```python
from build123d import *

# Parameters (mm, degrees)
F0_R     = 3.175
F1_DEPTH = 25.4
F2_R     = 2.38125
F3_DEPTH = 12.701
F4_SIZE2 = 0.79375
F4_SIZE  = 3.175


with BuildPart() as f1:
    # F0 (on Front) → F1 (new body)
    with BuildSketch(Plane.XZ):
        with BuildLine():
            ThreePointArc((6.35, 3.175), (3.175, -8.674261314), (11.849261314, 0))
            Line((11.849261314, 0), (228.6, 0))
            Line((228.6, 0), (228.6, 3.175))
            Line((228.6, 3.175), (6.35, 3.175))
        make_face()
        with Locations((6.35, -3.175)):
            Circle(F0_R, mode=Mode.SUBTRACT)
    extrude(amount=F1_DEPTH)

    # F2 (on face) → F3 (cut, through all)
    with BuildSketch(Plane.XY.offset(3.175)):
        with Locations((203.2, -12.7)):
            Circle(F2_R)
        with Locations((114.3, -12.7)):
            Circle(F2_R)
        with Locations((25.4, -12.7)):
            Circle(F2_R)
        Polygon((12.7, -8.382), (12.7, 5.4248190135), (-5.8604556464, 5.4248190135), (-5.8604556464, -32.8125189408), (12.7, -32.8125189408), (12.7, -16.764), (0, -16.764), (0, -8.382), align=None)
    extrude(amount=-F3_DEPTH, mode=Mode.SUBTRACT)

    # F4
    f4_edges = [f1.edges().sort_by_distance(p)[0] for p in [
        (120.65, -25.4, 0),
        (120.65, 0, 0),
        (228.6, -12.7, 0),
    ]]
    f4_side = f1.faces().sort_by_distance((120.570284, -12.699833, 0))[0]
    chamfer(f4_edges, length=F4_SIZE, length2=F4_SIZE2, reference=f4_side)


solid = f1.part
```
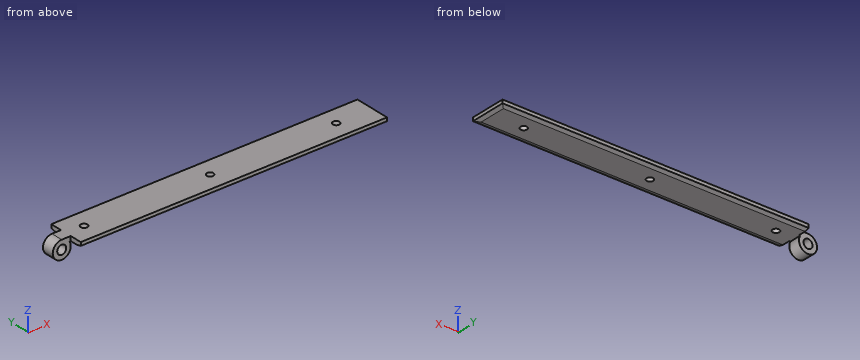
Geometry: final body of the model. Coordinates: model frame, mm. Coordinates: 2 decimals unless noted, no trailing zeros. Write each loop counter-clockwise with the first axis right and the second up, starting at its lowest first coordinate (ties: lowest second). Pieces come first, ordered by that corner, then holes. Notation, with made-up numbers: M 5.25,-23 L 48.25,-23 A16 ccw 48.25,4 Z; hole C 11,85.5 d3. An arc over 180 degrees is marked long. Answer as CSV lines item,"result". Start each with the question number.
Q1. Pin query (flat end, axial travel): P1, Ø7.5, axis at x = 6.35, z = -3.175, coming from the +Y side; P2, Ø1.5, axis at y = -4.5, z = -2.5, coming from the +X side; P3, Ø1, axis at y = -5, z = 2.5, coming from the -X side; P4, Ø8, axis at x = 183, y = -10.5, coming from the -Z side. Return the tip coordinate at first contact, or that it passes through.
Q2. Line query: line 1 (Z direction, x = 6.35, y = -12.25) (3 decimals); line 2 (Y direction, x = 114.3, z = 1.7); line 3 (X direction, y = -14, z = -3). Output: solid intervals per line, ascending. Write a range as from..to.
Q3. Cut plane A-A on y = -12.7. Return the cut outline in (x, z) (3 decimals), then the cut area to 3 significant figures.
Q4. Cut plane B-B on x = 203.2. Return the cut outline in (y, z) (3 decimals), then the cut area to 3 significant figures.
Q5. Cut plane C-C on x = 86. Return the cut outline in (y, z) (3 decimals).
Findings below:
1,P1,"stops at y = -8.38"
1,P2,"passes through"
1,P3,"stops at x = 12.7"
1,P4,"stops at z = 0"
2,line 1,"z = -9.525..-6.35, 0..3.175"
2,line 2,"y = -25.4..-15.08, -10.32..0"
2,line 3,"x = 0..3.18, 9.52..12.7"
3,outline,"M 6.35,3.175 A6.35 ccw long 11.849,0 L 23.019,0 L 23.019,3.175 Z; M 27.781,0 L 111.919,0 L 111.919,3.175 L 27.781,3.175 Z; M 116.681,0 L 200.819,0 L 200.819,3.175 L 116.681,3.175 Z; M 205.581,0 L 225.425,0 L 228.6,0.794 L 228.6,3.175 L 205.581,3.175 Z; hole C 6.35,-3.175 d6.35"
3,area,"742 mm2"
4,outline,"M -25.4,0.794 L -22.225,0 L -15.081,0 L -15.081,3.175 L -25.4,3.175 Z; M -10.319,0 L -3.175,0 L 0,0.794 L 0,3.175 L -10.319,3.175 Z"
4,area,"63.0 mm2"
5,outline,"M -25.4,0.794 L -22.225,0 L -3.175,0 L 0,0.794 L 0,3.175 L -25.4,3.175 Z"
